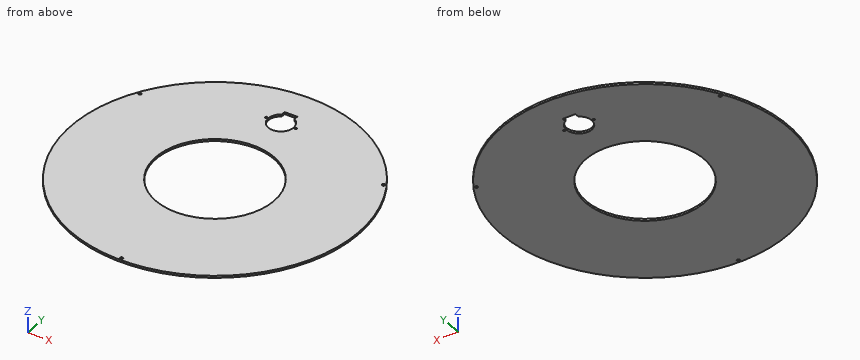
```python
from build123d import *

# Parameters (mm, degrees)
SCHIZZO1_R                   = 170
SCHIZZO1_R_2                 = 70
ESTRUSIONE_ESTRUSIONE1_DEPTH = 2.5
TAGLIO_ESTRUSIONE1_DEPTH     = 2.5
FORO_PER_VITE_M2_1_D         = 2.4
FORO_PER_VITE_M3_1_D         = 3.4
RIPETIZIONECIRCOLARE1_COUNT  = 3


with BuildPart() as part:
    # Schizzo1 → Estrusione-Estrusione1 (new body)
    with BuildSketch(Plane.XY):
        Circle(SCHIZZO1_R)
        Circle(SCHIZZO1_R_2, mode=Mode.SUBTRACT)
    extrude(amount=ESTRUSIONE_ESTRUSIONE1_DEPTH)

    # Schizzo3 → Taglio-Estrusione1 (cut)
    with BuildSketch(Plane.XY.offset(2.5)):
        with BuildLine():
            Line((7.5, 135.840381057), (-7.5, 135.840381057))
            Line((-7.5, 135.840381057), (-7.5, 130.840381057))
            ThreePointArc((-7.5, 130.840381057), (0, 102.85), (7.5, 130.840381057))
            Line((7.5, 130.840381057), (7.5, 135.840381057))
        make_face()
    extrude(amount=-TAGLIO_ESTRUSIONE1_DEPTH, mode=Mode.SUBTRACT)

    # Foro per Vite M2-1 (through all)
    with Locations(Plane.XY.offset(2.5)):
        with Locations((17.511664312, 117.848267331), (-17.511664312, 117.848267331)):
            Hole(FORO_PER_VITE_M2_1_D / 2)

    # Foro per Vite M3-1 (through all)
    with Locations(Plane.XY.offset(2.5)):
        with Locations((0, -166.830362559)):
            foro_per_vite_m3_1 = Hole(FORO_PER_VITE_M3_1_D / 2)

    # RipetizioneCircolare1: Foro per Vite M3-1 ×3 about axis
    ripetizionecircolare1_axis = Axis((0, 0, 0), (0, 0, 1))
    for i in range(1, RIPETIZIONECIRCOLARE1_COUNT):
        add(foro_per_vite_m3_1.rotate(ripetizionecircolare1_axis, i * 360 / RIPETIZIONECIRCOLARE1_COUNT), mode=Mode.SUBTRACT)


solid = part.part
```
Can you work these out from the model? Positions are in its coordinate system, mm. Give positions to 0.01 mm unless a question says otherwise; leave off trailing zeros. Loops run counter-clockwise (first coordinate to the right, second up) from the corner with the lowest first, then second, coordinate; pieces in that order, holes last. Notation, with made-up numbers: M 29,-9.75 L 44,-9.75 A19 cw 44,0.25 Z; hole C 74,67 d7. An arc over 180 degrees is marked long. Use one line per item in the form item = value. Start each with the question number.
(1) I want a section at B-B, the plane x = -49.5. Write out the boundary of the cut face in (y, z), and give its area (3 significant figures).
(2) I'm going to push flat-ended pins straight in: P1, Ø1, axis at y = 133.5, z = 0.5, coming from the +X side; P2, Ø1.2, axis at y = 133.5, z = 1, coming from the +X side; P3, Ø1, axis at x = 108.5, z = 0.5, coming from the -Y side. Where does each tip first touch, or does it pass through?
(3) Please list where these lines run through material, in increasing order: line 1 (Y direction, x = 0, z = 0.85); line 2 (Y direction, x = -12.5, z = 2.2); line 3 (Y direction, x = -24, z = 2.35).
(4) I want a section at C-C, the plane z = 1.4. Write out the boundary of the cut face in (x, y), and give its area (3 significant figures).
(5) I want a section at D-D, the plane x = -126.5. Write out the boundary of the cut face in (y, z).
(6) I want a section at A-A, the plane y = 0. Write out the boundary of the cut face in (x, z).
Worked out:
q1.outline = M -162.63,0 L -49.49,0 L -49.49,2.5 L -162.63,2.5 Z; M 49.49,0 L 162.63,0 L 162.63,2.5 L 49.49,2.5 Z
q1.area = 566 mm²
q2.P1 = 105.88
q2.P2 = 106.01
q2.P3 = -131.29
q3.line_1 = -170 to -168.53, -165.13 to -70, 70 to 102.85, 135.84 to 170
q3.line_2 = -169.54 to -68.87, 68.87 to 109.56, 126.14 to 169.54
q3.line_3 = -168.3 to -65.76, 65.76 to 168.3
q4.outline = C 0,0 d340; hole C -144.48,83.42 d3.4; hole C 0,0 d140; hole C -17.51,117.85 d2.4; hole M -7.5,130.84 A15 ccw long 7.5,130.84 L 7.5,135.84 L -7.5,135.84 Z; hole C 0,-166.83 d3.4; hole C 17.51,117.85 d2.4; hole C 144.48,83.42 d3.4
q4.area = 74,600 mm²
q5.outline = M -113.57,0 L 113.57,0 L 113.57,2.5 L -113.57,2.5 Z
q6.outline = M -170,0 L -70,0 L -70,2.5 L -170,2.5 Z; M 70,0 L 170,0 L 170,2.5 L 70,2.5 Z
